```python
from build123d import *

# Parameters (mm, degrees)
F0_W     = 76.2
F0_H     = 50.8
F1_DEPTH = 50.8
F2_SIZE  = 25.4
F3_R     = 12.7
F4_DEPTH = 50.8


with BuildPart() as f1:
    # F0 (on Front) → F1 (new body)
    with BuildSketch(Plane.XZ):
        with Locations((-38.1, 25.4)):
            Rectangle(F0_W, F0_H)
    extrude(amount=F1_DEPTH)

    # F2
    f2_edges = [f1.edges().sort_by_distance(p)[0] for p in [
        (0, -25.4, 50.8),
    ]]
    chamfer(f2_edges, length=F2_SIZE)

    # F3 (on face) → F4 (cut)
    with BuildSketch(Plane.XZ.offset(50.8)):
        with Locations((-25.4, 25.4)):
            Circle(F3_R)
    extrude(amount=-F4_DEPTH, mode=Mode.SUBTRACT)


solid = f1.part
```
Design review of the part built by this model. Coordinates are the model's own, in mm. Coordinates: 2 decimals unless noted, no trailing zeros. Write each loop counter-clockwise with the first axis right and the second up, starting at its lowest first coordinate (ties: lowest second). Pieces come first, ordered by that corner, then holes.
1) Add section D-D (x = -10). Write out the cut boundary in (y, z), plus the area to 3 significant figures.
2) Add section A-A (x = -31). Write out the cut boundary in (y, z), plus the area to 3 significant figures.
3) Mouldability with a two-part tool opening along Z and no side actions: class faces 1 (the flat face through (-47, 0, 26)), 2 (the cylindrical face through (-18.573, -25.756, 36.109)), 3 (the flat face through (-39, -25, 0)) as +Z half, -Z half, draft (parallel to the pull), parting line (faces both ways), or undercut.
4) Insertion check: pin 1 (4 mm diameter, centred on x = -37, z = 26, fed in from +Y); pin 2 (3 mm diameter, centred on y = -12.5, z = 38, fed in from +X); pin 3 (1 mm diameter, centred on x = -22, y = -26.5, fed in from +Z). Each pin has a flat end and moves straight along its axis. Give the tip position at first contact, or say it passes through.
5) Add section B-B (z = 14). Write out the cut boundary in (x, y).
6) Add section C-C (y = -19). Write out the cut boundary in (x, z), plus the area to 3 significant figures.
7) To check wall thickness, follow L1, parallel to Z at x = -25.4, y = -34; L2, parallel to X at y = -34, z = 25; L3, parallel to Z at x = -31, y = -30.5. State the ranges of each line that lie inside material, in increasing order.
Check result:
1. outline: (-50.8, 0) - (0, 0) - (0, 35.4) - (-50.8, 35.4) - close
1. area: 1,800 mm2
2. outline: (-50.8, 0) - (0, 0) - (0, 14) - (-50.8, 14) - close; (-50.8, 36.8) - (0, 36.8) - (0, 50.8) - (-50.8, 50.8) - close
2. area: 1,420 mm2
3. face 1: draft
3. face 2: undercut
3. face 3: -Z half
4. pin 1: stops at y = 0
4. pin 2: stops at x = -11.1
4. pin 3: stops at z = 47.9
5. outline: (-76.2, -50.8) - (-31, -50.8) - (-31, 0) - (-76.2, 0) - close; (-19.8, -50.8) - (0, -50.8) - (0, 0) - (-19.8, 0) - close
6. outline: (-76.2, 0) - (0, 0) - (0, 25.4) - (-25.4, 50.8) - (-76.2, 50.8) - close; hole circle Ø25.4 at (-25.4, 25.4)
6. area: 3,040 mm2
7. L1: z = 0 to 12.7, 38.1 to 50.8
7. L2: x = -76.2 to -38.09, -12.71 to 0
7. L3: z = 0 to 14, 36.8 to 50.8
